Input: dimensioned drawing with shaded views. Units: mm. Origin: part minimum x, y, z. Round coordinates to 2 decimals unless told otherwise and drop trailing zeros. Loops run counter-clockwise (first coordinate to the right, second up) from the corner with the lowest first, then second, coordinate; pieces in that order, holes last. Notation, with made-up numbers: M 29.5,48.25 L 34.5,48.25 A15 cw 34.5,62.25 Z; hole C 62,35.5 d2. An arc over 180 degrees is marked long. Answer as CSV lines item,"result". Start each with the question number.
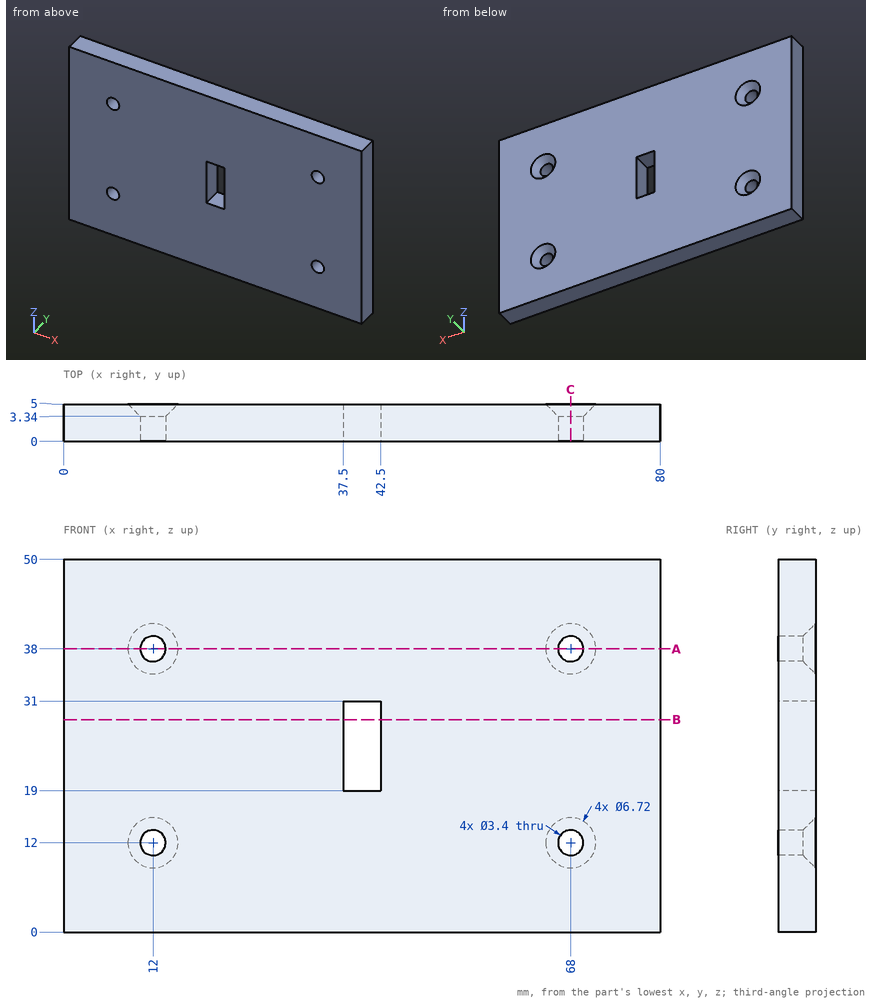
1) Section C-C, the plane x = 68. Return loops of the section in (y, z).
2) Section B-B, the plane z = 28.5. Return loops of the section in (x, y).
3) Ray query, line 1 along X through (y, z) = (1.85, 12); line 2 along Z through (x, y) = (68, 0.8); line 3 along Z through (x, y) = (67, 1.85). Return the intervals inside material, ascending.
4) Section A-A, the plane z = 38. Return loops of the section in (x, y).
5) Contact query for flat-ended pins moving along their axis: pin 1 Ø3 at (x, z) = (12, 38) entering from -Y; pin 2 Ø4.5 at (x, z) = (12, 12) entering from +Y. Output: stop coordinate, or through.
Findings below:
1,outline,"M 0,0 L 5,0 L 5,8.64 L 3.34,10.3 L 0,10.3 Z; M 0,13.7 L 3.34,13.7 L 5,15.36 L 5,34.64 L 3.34,36.3 L 0,36.3 Z; M 0,39.7 L 3.34,39.7 L 5,41.36 L 5,50 L 0,50 Z"
2,outline,"M 0,0 L 37.5,0 L 37.5,5 L 0,5 Z; M 42.5,0 L 80,0 L 80,5 L 42.5,5 Z"
3,line 1,"0 to 10.3, 13.7 to 66.3, 69.7 to 80"
3,line 2,"0 to 10.3, 13.7 to 36.3, 39.7 to 50"
3,line 3,"0 to 10.63, 13.37 to 36.63, 39.37 to 50"
4,outline,"M 0,0 L 10.3,0 L 10.3,3.34 L 8.64,5 L 0,5 Z; M 13.7,0 L 66.3,0 L 66.3,3.34 L 64.64,5 L 15.36,5 L 13.7,3.34 Z; M 69.7,0 L 80,0 L 80,5 L 71.36,5 L 69.7,3.34 Z"
5,pin 1,"through"
5,pin 2,"y = 3.89"
